Build history of the part. All positions in model axes, mm. Face numbers are marked on the shaded views. A direction names the side the tool comes from. Round coordinates to 2 decimals unless told otherwise and drop trailing zeros. Write each loop counter-clockwise with the first axis right and the second up, starting at its lowest first coordinate (ties: lowest second). Pieces come first, ordered by that corner, then holes. Notation, with made-up numbers: M -32.75,-29 L 9.25,-29 A6 cw 9.25,-18 Z; hole C -40,23.5 d9. An arc over 180 degrees is marked long. One line per item, written item: value. Start each with the question number.
```python
from build123d import *

# Parameters (mm, degrees)
SKETCH1_W                   = 22.6
SKETCH1_H                   = 12
BOSS_EXTRUDE1_DEPTH         = 3
BOSS_EXTRU_2_DEPTH          = 3
BOSS_EXTRU_1_REACH          = 45.022
ESQUISSE3_W                 = 8.636214684
ESQUISSE3_H                 = 11.84
ESQUISSE3_W_2               = 2.6
ENL_V_MAT_EXTRU_1_DEPTH     = 59.77153097
ESQUISSE6_R                 = 2
BOSS_EXTRU_3_DEPTH          = 17.7
ESQUISSE7_R                 = 1
ENL_V_MAT_EXTRU_3_DEPTH     = 4
R_VOLUTION1_ANGLE           = 90
R_VOLUTION1_OTHER_WAY_ANGLE = 90
REVOLVE1_ANGLE              = 30
REVOLVE1_OTHER_WAY_ANGLE    = 30
CONG_1_R                    = 3
CONG_2_R                    = 1
SKETCH3_W                   = 12.969079214
SKETCH3_H                   = 8.353445093
CUT_EXTRUDE1_DEPTH          = 11.84


with BuildPart() as part:
    # Sketch1 → Boss-Extrude1 (new body)
    with BuildSketch(Plane(origin=(0, 0, 0), x_dir=(1, 0, 0), z_dir=(0, 1, 0))):
        Polygon((33, 3), (33, 0), (0, 0), (0, 18), (33, 18), (33, 15), (31.6, 15), (31.6, 3), align=None)
        with Locations((15.8, 9)):
            Rectangle(SKETCH1_W, SKETCH1_H, mode=Mode.SUBTRACT)
    extrude(amount=BOSS_EXTRUDE1_DEPTH)

    # Esquisse4 → Boss.-Extru.2 (add)
    with BuildSketch(Plane.XZ):
        with BuildLine():
            Line((29.35, -17), (36.85, -18))
            Line((36.85, -18), (30.893033467, -21.572751002))
            ThreePointArc((30.893033467, -21.572751002), (29.35, -22), (27.806966533, -21.572751002))
            Line((27.806966533, -21.572751002), (21.85, -18))
            Line((21.85, -18), (29.35, -17))
        make_face()
        with BuildLine():
            Line((36.85, 0), (30.893033467, 3.572751002))
            ThreePointArc((30.893033467, 3.572751002), (29.35, 4), (27.806966533, 3.572751002))
            Line((27.806966533, 3.572751002), (21.85, 0))
            Line((21.85, 0), (29.35, -1))
            Line((29.35, -1), (36.85, 0))
        make_face()
    extrude(amount=-BOSS_EXTRU_2_DEPTH)

    # Boss.-Extru.1: up to this face of the body (flat: up to its plane)
    boss_extru_1_end = Plane(part.part.faces().sort_by_distance((10.925, 1.5, -18))[0])
    # Esquisse1 → Boss.-Extru.1 (add, up to the picked face)
    with BuildSketch(Plane.XY, mode=Mode.PRIVATE) as boss_extru_1_sk1:
        Polygon((43, -1), (33, 3), (28.66713547, 3), (28.66713547, 0), (38.66713547, -4), (54.04713547, -4), (54.04713547, -1), align=None)
    boss_extru_1_tool1 = split(extrude(boss_extru_1_sk1.sketch, amount=-BOSS_EXTRU_1_REACH, mode=Mode.PRIVATE), bisect_by=boss_extru_1_end, keep=Keep.BOTH, mode=Mode.PRIVATE)
    add(boss_extru_1_tool1.solids().sort_by(Axis((40.332957, -1.209124, 0), (0, 0, -1)))[0])

    # Esquisse3 → Enlèv. mat.-Extru.1 (cut, through all)
    with BuildSketch(Plane.XZ.offset(4)):
        with Locations((34.349028128, -9)):
            Rectangle(ESQUISSE3_W, ESQUISSE3_H)
        with Locations((49.115, -9)):
            Rectangle(ESQUISSE3_W_2, ESQUISSE3_H)
    extrude(amount=-ENL_V_MAT_EXTRU_1_DEPTH, mode=Mode.SUBTRACT)

    # Esquisse6 → Boss.-Extru.3 (add)
    with BuildSketch(Plane(origin=(0, 3, 0), x_dir=(1, 0, 0), z_dir=(0, 1, 0))):
        with Locations(Location((29.35, -1, 0), (0, 0, 90))):
            Circle(ESQUISSE6_R)
        with Locations(Location((29.35, 19, 0), (0, 0, 270))):
            Circle(ESQUISSE6_R)
    extrude(amount=BOSS_EXTRU_3_DEPTH)

    # Esquisse7 → Enlèv. mat.-Extru.3 (cut)
    with BuildSketch(Plane(origin=(0, 20.7, 0), x_dir=(1, 0, 0), z_dir=(0, 1, 0))):
        with Locations(Location((29.35, 19, 0), (0, 0, 270))):
            Circle(ESQUISSE7_R)
        with Locations(Location((29.35, -1, 0), (0, 0, 270))):
            Circle(ESQUISSE7_R)
    extrude(amount=-ENL_V_MAT_EXTRU_3_DEPTH, mode=Mode.SUBTRACT)



with BuildPart() as body_2:
    # Esquisse8 → Révolution1 (revolve)
    with BuildSketch(Plane.XY.offset(-9)):
        Polygon((56.665, -9.36), (54.165, -9.36), (54.165, -11.86), (59.165, -11.86), (59.165, -7.16), (56.665, -7.16), align=None)
    revolve(axis=Axis((74.438744763, 4.84, -9), (1, 0, 0)), revolution_arc=R_VOLUTION1_ANGLE)

    # Esquisse8 → Révolution1 other way (revolve)
    with BuildSketch(Plane.XY.offset(-9)):
        Polygon((56.665, -9.36), (54.165, -9.36), (54.165, -11.86), (59.165, -11.86), (59.165, -7.16), (56.665, -7.16), align=None)
    revolve(axis=Axis((74.438744763, 4.84, -9), (-1, 0, 0)), revolution_arc=R_VOLUTION1_OTHER_WAY_ANGLE)


with BuildPart() as part_1:
    add(part.part)

    add(body_2.part)  # Revolve1 merges body 2
    # Esquisse8<5> → Revolve1 (revolve)
    with BuildSketch(Plane.XY.offset(-9)):
        Polygon((54.165, -11.86), (54.165, -9.36), (54.165, -4), (51.665, -4), (51.665, -11.86), align=None)
    revolve(axis=Axis((74.438744763, 4.84, -9), (1, 0, 0)), revolution_arc=REVOLVE1_ANGLE)

    # Esquisse8<5> → Revolve1 other way (revolve)
    with BuildSketch(Plane.XY.offset(-9)):
        Polygon((54.165, -11.86), (54.165, -9.36), (54.165, -4), (51.665, -4), (51.665, -11.86), align=None)
    revolve(axis=Axis((74.438744763, 4.84, -9), (-1, 0, 0)), revolution_arc=REVOLVE1_OTHER_WAY_ANGLE)

    # Congé1
    cong_1_edges = [part_1.edges().sort_by_distance(p)[0] for p in [
        (0, 1.5, -18),
        (0, 1.5, 0),
    ]]
    fillet(cong_1_edges, radius=CONG_1_R)

    # Congé2
    cong_2_edges = [part_1.edges().sort_by_distance(p)[0] for p in [
        (59.165, -11.86, -9),
    ]]
    fillet(cong_2_edges, radius=CONG_2_R)

    # Sketch3 → Cut-Extrude1 (cut)
    with BuildSketch(Plane.XY.offset(-14.92)):
        with Locations((36.515460393, 3.176722547)):
            Rectangle(SKETCH3_W, SKETCH3_H)
    extrude(amount=CUT_EXTRUDE1_DEPTH, mode=Mode.SUBTRACT)


solid = part_1.part
```
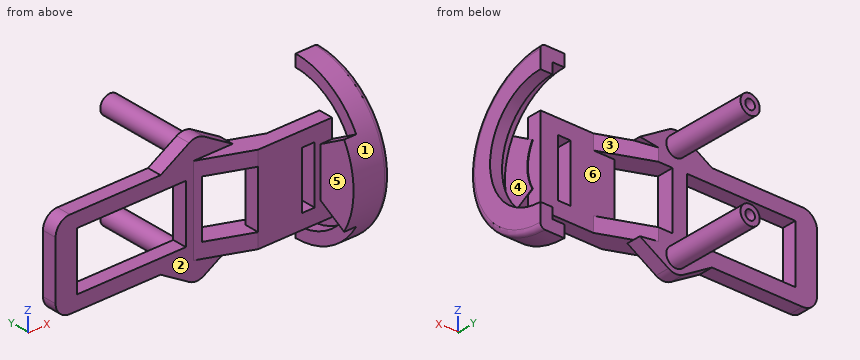
Item 1: Two-plate mould, pull along Z, no slides. Class the marked faces 1, 2 and 3: pulls with the +Z half, pulls with the -Z half, needs draft (parallel to the pull), parting line crosses it, or undercut.
Item 2: Drill centre lines: line 1 (X direction, y = 18.35, z = 1); line 2 (Z direction, x = 29, y = 18); line 3 (Y direction, x = 3, z = -5). Where is each one in solid material? Low to high.
Item 3: Cut at D-D, the plane y = 4. Count the separate pieces of the cut face and the enclosed holes in it, plus the area to 3 significant figures.
Item 4: Cut at C-C, the plane x = 23.5. Write the cut outline in (y, z).
Item 5: Cut at B-B, the plane z = -9. Write the cut outline in (x, y) (3 decimals), plus the area to 3 significant figures.
Item 6: Cut at A-A, the plane x = 14. Write the cut outline in (y, z), plus the area to 3 significant figures.
Item 7: Which spindle directions (+Z, -Z, +X, -X, +Y, -Y) get a long thin tool onto all of the face, cutting with end or side? Do the marked faces 4, 5 and 6. Say none if no direction does.
Item 8: Drop flat-ended pins along their axis: pin 1 (4 mm diameter, centred on y = -1, z = -13, fed in from +X) (3 decimals); pin 2 (5 mm diameter, centred on y = -5.5, z = 5, fed in from -X) (3 decimals); pin 3 (3.5 mm diameter, centred on x = 16.5, y = 2, fed in from -Z); pin 4 (10 mm diameter, centred on x = 26.5, y = -7.5, fed in from +Z). Give the stop position or say it passes through.
Computed values:
1. face 1: parting line crosses it
1. face 2: needs draft
1. face 3: undercut
2. line 1: x = 27.35 to 28.35, 30.35 to 31.35
2. line 2: z = -20.97 to -19.94, -18.06 to -17.03, -0.97 to 0.06, 1.94 to 2.97
2. line 3: y = 0 to 3
3. separate pieces: 4
3. enclosed holes: 0
3. area: 60.8 mm2
4. outline: M 0,-18.99 L 3,-18.99 L 3,-15 L 0,-15 Z; M 0,-3 L 3,-3 L 3,0.99 L 0,0.99 Z
5. outline: M 0,0 L 4.5,0 L 4.5,3 L 0,3 Z; M 27.1,0 L 28.667,0 L 30.031,-0.546 L 30.031,3 L 27.1,3 Z; M 38.667,-4 L 47.815,-4 L 47.815,-1 L 38.667,-1 Z; M 50.415,-4 L 51.665,-4 L 51.665,-11.86 L 58.165,-11.86 A1 ccw 59.165,-10.86 L 59.165,-7.16 L 56.665,-7.16 L 56.665,-9.36 L 54.165,-9.36 L 54.165,-4 L 54.047,-4 L 54.047,-1 L 50.415,-1 Z
5. area: 98.4 mm2
6. outline: M 0,-18 L 3,-18 L 3,-15 L 0,-15 Z; M 0,-3 L 3,-3 L 3,0 L 0,0 Z
6. area: 18.0 mm2
7. face 4: +Y
7. face 5: +Z, -Z, -X, -Y
7. face 6: +X, +Y
8. pin 1: stops at x = 54.165
8. pin 2: stops at x = 54.165
8. pin 3: stops at z = -18
8. pin 4: passes through
